from build123d import *

# Parameters (mm, degrees)
CHAMFER1_SIZE = 0.5


with BuildPart() as part:
    # Sketch1 → Revolve1 (revolve)
    with BuildSketch(Plane.XY):
        Polygon((0, 0), (92, 0), (92, -5), (90.1, -5), (90.1, -2), (84.9, -2), (84.9, -5), (83, -5), (83, -1.2), (0, -1.2), align=None)
    revolve(axis=Axis((0, -1.2, 0), (0, 1, 0)))

    # Chamfer1
    chamfer1_edges = [part.edges().sort_by_distance(p)[0] for p in [
        (-92, -5, 0),
        (-92, 0, 0),
        (-83, -1.2, 0),
        (-83, -5, 0),
        (-84.9, -5, 0),
        (-90.1, -5, 0),
    ]]
    chamfer(chamfer1_edges, length=CHAMFER1_SIZE)


solid = part.part
Design review of the part built by this model. Coordinates are the model's own, in mm. A direction names the side the tool comes from. Give positions to 0.01 mm unless a question says otherwise; leave off trailing zeros. Loops run counter-clockwise (first coordinate to the right, second up) from the corner with the lowest first, then second, coordinate; pieces in that order, holes last. Notation, with made-up numbers: (-1, 21.5) - (25, 21.5) arc R9 cw to (25, 34.5) - close; hole circle Ø5 at (-35.5, 75.25). An arc over 180 degrees is marked (long way). Write item = value, one per line.
1) Take a section at B-B on x = 0. State the section outline as (y, z) points, and give its area (3 significant figures).
Result sheet:
outline = (-5, -91.5) - (-4.5, -92) - (-0.5, -92) - (0, -91.5) - (0, 91.5) - (-0.5, 92) - (-4.5, 92) - (-5, 91.5) - (-5, 90.6) - (-4.5, 90.1) - (-2, 90.1) - (-2, 84.9) - (-4.5, 84.9) - (-5, 84.4) - (-5, 83.5) - (-4.5, 83) - (-1.7, 83) - (-1.2, 82.5) - (-1.2, -82.5) - (-1.7, -83) - (-4.5, -83) - (-5, -83.5) - (-5, -84.4) - (-4.5, -84.9) - (-2, -84.9) - (-2, -90.1) - (-4.5, -90.1) - (-5, -90.6) - close
area = 257 mm2
2) Take a section at A-A on y = -3.4. State the section outline as (x, z) points.
Result sheet:
outline = circle Ø184 at (0, 0); circle Ø169.8 at (0, 0); hole circle Ø180.2 at (0, 0); hole circle Ø166 at (0, 0)
3) To check wall thickness, follow line 1 (X direction, y = -3.75, z = 0); line 2 (X direction, y = -2.95, z = -23.5). State the ranges of each line that lie inside material, in increasing order.
Result sheet:
line_1 = -92 to -90.1, -84.9 to -83, 83 to 84.9, 90.1 to 92
line_2 = -88.95 to -86.98, -81.58 to -79.6, 79.6 to 81.58, 86.98 to 88.95
4) Clearance check with flat-ended pins moving along their axes: pin 1 Ø3 at (y, z) = (-1, 23.5) entering from -X; pin 2 Ø5 at (x, z) = (33.5, -67) entering from +Y; pin 3 Ø12 at (x, z) = (20.5, -58.5) entering from -Y; pin 4 Ø3 at (y, z) = (-2.5, 22) entering from -X. State where each tip first meets the part, or that it passes through.
Result sheet:
pin_1 = -89.33
pin_2 = 0
pin_3 = -1.2
pin_4 = -89.69
5) Take a section at C-C on z = 0. State the section outline as (x, y) points.
Result sheet:
outline = (-92, -4.5) - (-91.5, -5) - (-90.6, -5) - (-90.1, -4.5) - (-90.1, -2) - (-84.9, -2) - (-84.9, -4.5) - (-84.4, -5) - (-83.5, -5) - (-83, -4.5) - (-83, -1.7) - (-82.5, -1.2) - (82.5, -1.2) - (83, -1.7) - (83, -4.5) - (83.5, -5) - (84.4, -5) - (84.9, -4.5) - (84.9, -2) - (90.1, -2) - (90.1, -4.5) - (90.6, -5) - (91.5, -5) - (92, -4.5) - (92, -0.5) - (91.5, 0) - (-91.5, 0) - (-92, -0.5) - close
6) Draft analysis for pull direction X (two halves, no side actions). For faces 1 (the face through (79.167, -3.08, -24.931)), 2 (the face through (-19, -5, -82)), 3 (the face through (-11.977, -2.528, -91.217)), state which applies: +X half, -X half, draft (parallel to the pull), parting line (faces both ways), or undercut.
Result sheet:
face_1 = undercut
face_2 = draft
face_3 = parting line
7) Tool access review of faces 4 (the face through (1, 0, -1)), 5 (the face through (48.44, -3.23, -75.97)): name each direction out of +Z, -Z, +X, -X, +Y, -Y from which nothing blocks a thin tool from reaching the whole face with its end or side.
Result sheet:
face_4 = +Z, -Z, +X, -X, +Y
face_5 = -Y
